Input: part model. Units: mm. Frame: model coordinates. Coordinates: 2 decimals unless noted, no trailing zeros. Write each loop counter-clockwise with the first axis right and the second up, starting at its lowest first coordinate (ties: lowest second). Pieces come first, ordered by that corner, then holes.
1) Section query A-A (y = 30). Output: boundary loops of the cut face in (x, z).
2) Section query B-B (x = -21.5). Output: boundary loops of the cut face in (y, z).
3) Pin query (flat end, axial travel): pin 1 Ø3.5 at (x, y) = (-32.89, 32.89) entering from +Z. Return the tip coordinate at first contact, or that it passes through.
4) Line query: L1, parallel to Y at x = -32.89, z = 42.05; L2, parallel to Y at x = 27, z = 41.65; L3, parallel to X at y = 29.5, z = 42.25. Output: solid intervals per line, ascending.
from build123d import *

# Parameters (mm, degrees)
SKETCH019_W     = 72.78
SKETCH019_H     = 72.78
PAD009_DEPTH    = 3
SKETCH040_R     = 1.5
POCKET007_DEPTH = 3.001
SKETCH046_R     = 1.5
POCKET008_DEPTH = 3.001
SKETCH079_R     = 1.25
POCKET016_DEPTH = 3.001


with BuildPart() as part:
    # Sketch019 → Pad009 (new body)
    with BuildSketch(Plane.XY):
        Rectangle(SKETCH019_W, SKETCH019_H)
    extrude(amount=PAD009_DEPTH)

    # Sketch040 → Pocket007 (cut, through all)
    with BuildSketch(Plane.XY.offset(3)):
        with Locations((-32.89, 32.89)):
            Circle(SKETCH040_R)
        with Locations((32.89, 32.89)):
            Circle(SKETCH040_R)
        with Locations((-32.89, -32.89)):
            Circle(SKETCH040_R)
        with Locations((32.89, -32.89)):
            Circle(SKETCH040_R)
    extrude(amount=-POCKET007_DEPTH, mode=Mode.SUBTRACT)

    # Sketch046 (on Face5 of Pocket007) → Pocket008 (cut, through all)
    with BuildSketch(Plane.XY.offset(3)):
        with Locations((-3, 30)):
            Circle(SKETCH046_R)
        with Locations((27, 30)):
            Circle(SKETCH046_R)
        with Locations((-3, -32)):
            Circle(SKETCH046_R)
        with Locations((27, -32)):
            Circle(SKETCH046_R)
    extrude(amount=-POCKET008_DEPTH, mode=Mode.SUBTRACT)

    # Sketch079 (on Face5 of Pocket008) → Pocket016 (cut, through all)
    with BuildSketch(Plane.XY.offset(3)):
        with Locations((-21.5, 34.75)):
            Circle(SKETCH079_R)
        with Locations((-8.5, 34.75)):
            Circle(SKETCH079_R)
        with Locations((-21.5, -34.75)):
            Circle(SKETCH079_R)
        with Locations((-8.5, -34.75)):
            Circle(SKETCH079_R)
    extrude(amount=-POCKET016_DEPTH, mode=Mode.SUBTRACT)


with BuildPart() as part_1:
    # Body002 placement: moved
    add(part.part.moved(Location((0, 0, 41))))


solid = part_1.part
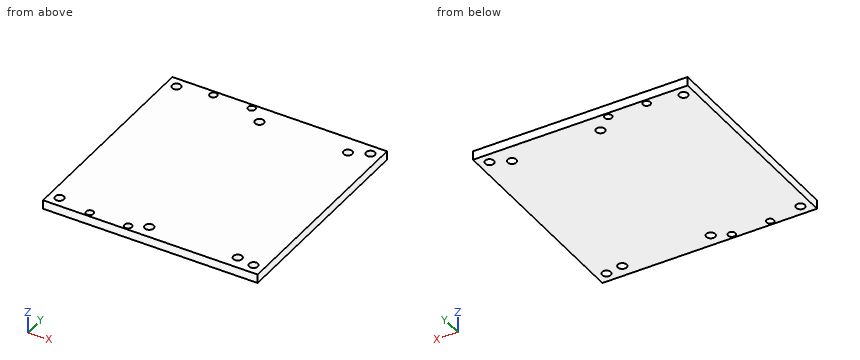
Answer:
1. outline: (-36.39, 41) - (-4.5, 41) - (-4.5, 44) - (-36.39, 44) - close; (-1.5, 41) - (25.5, 41) - (25.5, 44) - (-1.5, 44) - close; (28.5, 41) - (36.39, 41) - (36.39, 44) - (28.5, 44) - close
2. outline: (-36.39, 41) - (-36, 41) - (-36, 44) - (-36.39, 44) - close; (-33.5, 41) - (33.5, 41) - (33.5, 44) - (-33.5, 44) - close; (36, 41) - (36.39, 41) - (36.39, 44) - (36, 44) - close
3. pin 1: stops at z = 44
4. L1: y = -36.39 to -34.39, -31.39 to 31.39, 34.39 to 36.39
4. L2: y = -36.39 to -33.5, -30.5 to 28.5, 31.5 to 36.39
4. L3: x = -36.39 to -4.41, -1.59 to 25.59, 28.41 to 36.39
